```python
from build123d import *
from build123d.topology import SkipClean

# Parameters (mm, degrees)
BOSS_EXTRUDE1_DEPTH = 13
SKETCH2_W           = 5
SKETCH2_H           = 8
CUT_EXTRUDE1_DEPTH  = 21.383817111
SKETCH3_R           = 1.55
CUT_EXTRUDE2_DEPTH  = 21.383817111
FILLET1_R           = 1
FILLET2_R           = 2.5
CHAMFER1_SIZE       = 4
FILLET3_R           = 2.25
FILLET4_R           = 2.25
CHAMFER2_START      = -13
CHAMFER2_DEPTH      = 13
CHAMFER2_START_2    = -5
CHAMFER2_2_DEPTH    = 5
CHAMFER2_START_3    = -8
CHAMFER2_3_DEPTH    = 1.181980515


with BuildPart() as part:
    # Sketch1 → Boss-Extrude1 (new body)
    with BuildSketch(Plane.XY):
        Polygon((6, 0), (-6, 0), (-6, -9.5), (-12.5, -9.5), (-12.5, -8), (-7.5, -8), (-7.5, 1.5), (7.5, 1.5), (7.5, -8), (12.5, -8), (12.5, -9.5), (6, -9.5), align=None)
    extrude(amount=-BOSS_EXTRUDE1_DEPTH)

    # Sketch2 → Cut-Extrude1 (cut, through all)
    with BuildSketch(Plane(origin=(0, -8, 0), x_dir=(1, 0, 0), z_dir=(0, 1, 0))):
        with Locations((10, 9)):
            Rectangle(SKETCH2_W, SKETCH2_H)
    extrude(amount=-CUT_EXTRUDE1_DEPTH, mode=Mode.SUBTRACT)

    # Sketch3 → Cut-Extrude2 (cut, through all)
    with BuildSketch(Plane(origin=(0, -8, 0), x_dir=(1, 0, 0), z_dir=(0, 1, 0))):
        with Locations(Location((10, 2.5, 0), (0, 0, 180))):
            Circle(SKETCH3_R)
        with Locations(Location((-10, 2.5, 0), (0, 0, 180))):
            Circle(SKETCH3_R)
    extrude(amount=-CUT_EXTRUDE2_DEPTH, mode=Mode.SUBTRACT)

    # Fillet1
    fillet1_edges = [part.edges().sort_by_distance(p)[0] for p in [
        (6, 0, -6.5),
        (-6, 0, -6.5),
    ]]
    fillet(fillet1_edges, radius=FILLET1_R)

    # Fillet2
    fillet2_edges = [part.edges().sort_by_distance(p)[0] for p in [
        (-7.5, 1.5, -6.5),
        (7.5, 1.5, -6.5),
    ]]
    fillet(fillet2_edges, radius=FILLET2_R)

    # Chamfer1
    chamfer1_edges = [part.edges().sort_by_distance(p)[0] for p in [
        (-12.5, -8.75, -13),
    ]]
    chamfer(chamfer1_edges, length=CHAMFER1_SIZE)

    # Fillet3
    fillet3_edges = [part.edges().sort_by_distance(p)[0] for p in [
        (-12.5, -8.75, -9),
        (-8.5, -8.75, -13),
    ]]
    fillet(fillet3_edges, radius=FILLET3_R)

    # Fillet4
    fillet4_edges = [part.edges().sort_by_distance(p)[0] for p in [
        (12.5, -8.75, -5),
    ]]
    fillet(fillet4_edges, radius=FILLET4_R)

    # Chamfer2: read off the stored shape, not the designer's step
    # Chamfer2 outline → Chamfer2 (add)
    with BuildSketch(Plane.XY.offset(CHAMFER2_START)):
        Polygon((-7.5, -8), (-7.5, -6.75), (-8.75, -8), align=None)
    extrude(amount=CHAMFER2_DEPTH)

    # Chamfer2 2 outline → Chamfer2 2 (add)
    with BuildSketch(Plane.XY.offset(CHAMFER2_START_2)):
        Polygon((7.5, -8), (8.75, -8), (7.5, -6.75), align=None)
    extrude(amount=CHAMFER2_2_DEPTH)

    # Chamfer2 3 outline → Chamfer2 3 (cut)
    with SkipClean():  # the faces are left unmerged after this step: merging them gives an invalid solid
        with BuildSketch(Plane(origin=(0, 0, 0), x_dir=(1, 0, 0), z_dir=(0, 1, 0)).offset(CHAMFER2_START_3)):
            with BuildLine():
                Line((8.75, 1.583484861), (8.75, 3.416515139))
                ThreePointArc((8.75, 3.416515139), (8.45, 2.5), (8.75, 1.583484861))
            make_face()
            with BuildLine():
                Line((-7.568019485, 13), (-8.75, 13))
                Line((-8.75, 13), (-8.75, 12.664529201))
                ThreePointArc((-8.75, 12.664529201), (-8.182352171, 12.914508108), (-7.568019485, 13))
            make_face()
            with BuildLine():
                ThreePointArc((-8.75, 1.583484861), (-8.45, 2.5), (-8.75, 3.416515139))
                Line((-8.75, 3.416515139), (-8.75, 1.583484861))
            make_face()
        extrude(amount=CHAMFER2_3_DEPTH, mode=Mode.SUBTRACT)


solid = part.part
```
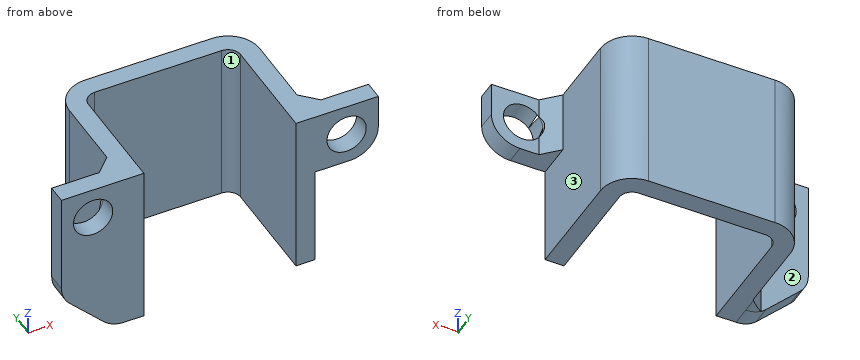
Source: CAD feature listing. Evaluate the final solid. Frame: model axes, mm. Face numbers are marked on the shaded views. A direction names the side the tool comes from. Give positions to 0.01 mm unless a question says otherwise; leave off trailing zeros. Loops run counter-clockwise (first coordinate to the right, second up) from the corner with the lowest first, then second, coordinate; pieces in that order, holes last. Notation, with made-up numbers: (-4, 11) -> (9, 11) arc R12 cw to (9, 26) -> close; hole circle Ø2 at (-32, -23.75). An arc over 180 degrees is marked (long way). Put each result on its own line as item: value. Start each with the question number.
1) Cut plane C-C (z = -3.75). Return loops of the section in (x, y), then the cut area to 3 significant figures.
2) Cut plane B-B (y = -6.5). Return loops of the section in (x, z).
3) Material intervals for probe 1 along X at (y, z) = (-9.05, -2.5); probe 2 along X at (y, z) = (-2.5, -2); probe 3 along Z at (x, y) = (10, -9.1), sorted ascending.
4) Reachability of the marked faces 1, 2 and 3 from +Z, -Z, +X, -X, +Y, -Y: full face, straight path, thin tool, end or side. Return the list, or none.
5) Contact query for flat-ended pins moving along their axis: P1, Ø1.5, axis at y = -8, z = -6, coming from the +X side; P2, Ø3, axis at x = -0.5, z = -4.5, coming from the -Y side; P3, Ø3, axis at y = -4.5, z = -6.5, coming from the -X side. Output: stop coordinate, or through.
6) Cut plane A-A (x = -10). Return loops of the section in (y, z).
7) Cut plane D-D (z = -12). Return loops of the section in (x, y).
Results are:
1. outline: (-12.5, -9.5) -> (-10.92, -9.5) -> (-10.92, -8) -> (-12.5, -8) -> close; (-9.08, -9.5) -> (-6, -9.5) -> (-6, -1) arc R1 cw to (-5, 0) -> (5, 0) arc R1 cw to (6, -1) -> (6, -9.5) -> (9.08, -9.5) -> (9.08, -8) -> (8.75, -8) -> (7.5, -6.75) -> (7.5, -1) arc R2.5 ccw to (5, 1.5) -> (-5, 1.5) arc R2.5 ccw to (-7.5, -1) -> (-7.5, -6.75) -> (-8.75, -8) -> (-9.08, -8) -> close; (10.92, -9.5) -> (12.27, -9.5) -> (12.27, -8) -> (10.92, -8) -> close
1. area: 59.5 mm2
2. outline: (-7.5, -13) -> (-6, -13) -> (-6, 0) -> (-7.5, 0) -> close; (6, -13) -> (7.5, -13) -> (7.5, 0) -> (6, 0) -> close
3. probe 1: x = -12.5 to -11.55, -8.45 to -6, 6 to 8.45, 11.55 to 12.5
3. probe 2: x = -7.5 to -6, 6 to 7.5
3. probe 3: z = -5 to -4.05, -0.95 to 0
4. face 1: +Z, -Z, -Y
4. face 2: +Z, -Z, -X, +Y
4. face 3: -Z, +X, +Y
5. P1: stops at x = 7.5
5. P2: stops at y = 0
5. P3: stops at x = -7.5
6. outline: (-9.5, -11.5) -> (-8, -11.5) -> (-8, -4.05) -> (-9.5, -4.05) -> close; (-9.5, -0.95) -> (-8, -0.95) -> (-8, 0) -> (-9.5, 0) -> close
7. outline: (-9.5, -9.5) -> (-6, -9.5) -> (-6, -1) arc R1 cw to (-5, 0) -> (5, 0) arc R1 cw to (6, -1) -> (6, -9.5) -> (7.5, -9.5) -> (7.5, -1) arc R2.5 ccw to (5, 1.5) -> (-5, 1.5) arc R2.5 ccw to (-7.5, -1) -> (-7.5, -6.75) -> (-8.75, -8) -> (-9.5, -8) -> close
